The drawing under review shows one solid part. Ordinate dimensions are in mm from its lowest x, y, z. Give positions to 0.01 mm unless a question says otherwise; leave off trailing zeros. Order: outer loops, then holes, each group sorted by start corner. A loop starts at its lowest first (then second) coordinate and runs counter-clockwise, first axis right, second up. Notation, with made-up numbers: (56.25, -40) - (98.25, -40) arc R31 cw to (98.25, -13) - close; hole circle Ø2 at (53.5, 60.5). An arc over 180 degrees is marked (long way). Answer as a JSON object with one key per item and string values. Group by question number.
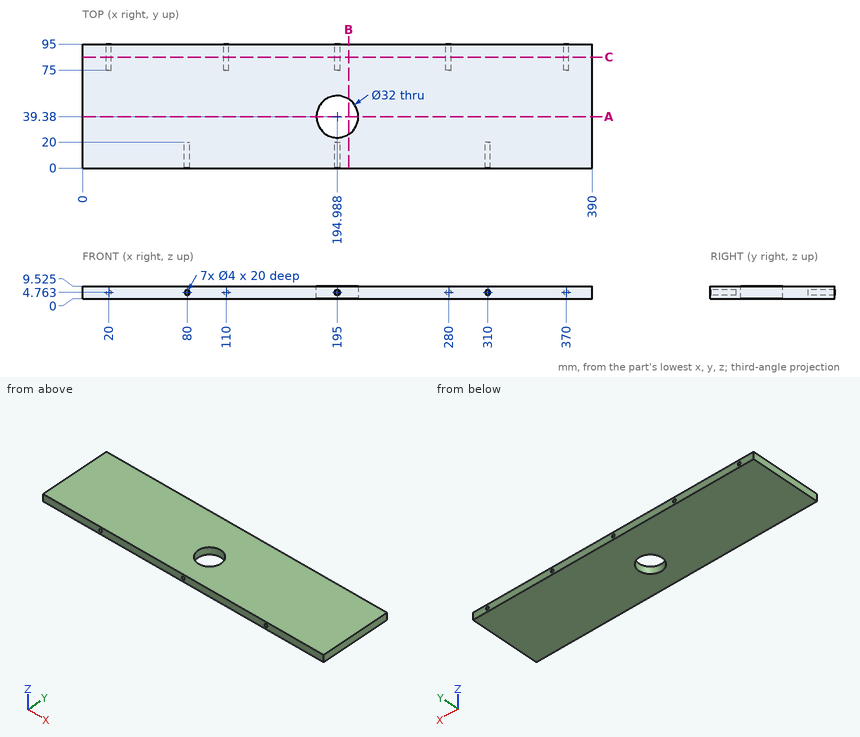
1) For line 1 (X direction, y = 83.5, z = 5.25); line 2 (Z direction, x = 195, y = 7.75) (1 decimal); line 3 (X direction, y = 42, z = 0.5) (1 decimal), list the stretches that pass through material, from the lowest coordinate up.
2) Consider section C-C (y = 85). Give the boundary of the cut face in (x, z) (1 decimal), plus the area to 3 significant figures.
3) Consider section B-B (x = 203.5). Give the boundary of the cut face in (y, z) (1 decimal).
4) Consider section A-A (y = 39.38). Give the boundary of the cut face in (x, z) (1 decimal).
5) For pin 1 (5 mm diameter, centred on x = 20, z = 4.76, fed in from -Y); pin 2 (2 mm diameter, centred on x = 195, z = 4, fed in from +Y); pin 3 (1.2 mm diameter, centred on x = 310.5, z = 4.5, fed in from -Y), all flat-tipped, find the tip position at first contact; note any pin that passes through.
Result set:
{
 "1": {"line 1": "x = 0 to 18.06, 21.94 to 108.06, 111.94 to 193.06, 196.94 to 278.06, 281.94 to 368.06, 371.94 to 390", "line 2": "z = 0 to 2.8, 6.8 to 9.5", "line 3": "x = 0 to 179.2, 210.8 to 390"},
 "2": {"outline": "(0, 0) - (390, 0) - (390, 9.5) - (0, 9.5) - close; hole circle Ø4 at (20, 4.8); hole circle Ø4 at (110, 4.8); hole circle Ø4 at (195, 4.8); hole circle Ø4 at (280, 4.8); hole circle Ø4 at (370, 4.8)", "area": "3,650 mm2"},
 "3": {"outline": "(0, 0) - (25.8, 0) - (25.8, 9.5) - (0, 9.5) - close; (52.9, 0) - (95, 0) - (95, 9.5) - (52.9, 9.5) - close"},
 "4": {"outline": "(0, 0) - (179, 0) - (179, 9.5) - (0, 9.5) - close; (211, 0) - (390, 0) - (390, 9.5) - (211, 9.5) - close"},
 "5": {"pin 1": "stops at y = 0", "pin 2": "stops at y = 75", "pin 3": "stops at y = 20"}
}
